Geometry: final body of the model. Coordinates: model frame, mm. A direction names the side the tool comes from. Round coordinates to 2 decimals unless told otherwise and drop trailing zeros. Loops run counter-clockwise (first coordinate to the right, second up) from the corner with the lowest first, then second, coordinate; pieces in that order, holes last. Notation, with made-up numbers: M 76.5,29 L 130.5,29 A15 ccw 130.5,57 Z; hole C 71,58 d4. An arc over 180 degrees is marked long. Answer as a JSON object with one key per item and string values.
Autodesk Fusion 360 part; units mm, degrees
sketch "Sketch1" plane through (0, 0, 0) normal (0, 0, 1) x (1, 0, 0)
  line L0 (7, -22) -> (-7, -22)
  line L1 (-7, -22) -> (-7, 22)
  line L2 (-7, 22) -> (7, 22)
  line L3 (7, 22) -> (7, -22)
  line L4 (7, -22) -> (-7, 22) construction
  line L5 (-7, -22) -> (7, 22) construction
  circle A0 centre (0, 0) radius 3.2483
  circle A1 centre (0, 16) radius 0.75
  circle A2 centre (0, -16) radius 0.75
  dimension "d1" = 1.5
  dimension "d2" = 1.5
extrude "Extrude1" add sketch "Sketch1" along normal blind 13
extrude "Extrude2" add 1 faces at (-2.3333, 22, 4.3333) along direction (0, 1, 0) blind 6
extrude "Extrude3" add 1 faces at (2.3333, -22, 4.3333) along direction (0, -1, 0) blind 6
sketch "Sketch2" plane through (0, 0, 13) normal (0, 0, 1) x (-1, 0, 0)
  circle A0 centre (0, 0) radius 3.2483
  circle A1 centre (0, 16) radius 0.75
  circle A2 centre (0, -16) radius 0.75
  line L0 (7, -28) -> (7, 28)
  line L1 (7, 28) -> (-7, 28)
  line L2 (-7, 28) -> (-7, -28)
  line L3 (-7, -28) -> (7, -28)
sketch "Sketch3" plane through (0, 0, 13) normal (0, 0, 1) x (-1, 0, 0)
  line L0 (7, -28) -> (-7, -28)
  line L1 (-7, -28) -> (-7, -20)
  line L2 (-7, -20) -> (7, -20)
  line L3 (7, -20) -> (7, -28)
  line L4 (7, 20) -> (-7, 20)
  line L5 (-7, 20) -> (-7, 28)
  line L6 (-7, 28) -> (7, 28)
  line L7 (7, 28) -> (7, 20)
extrude "Extrude4" add sketch "Sketch3" along normal blind 11
extrude "Extrude5" add 2 faces at (-2.3333, 25.3333, 24) (-2.3333, -22.6667, 24) along direction (0, 0, 1) blind 9.65
sketch "Sketch4" plane through (7, 0, 0) normal (1, 0, 0) x (0, 1, 0)
  line L0 (-28, 0) -> (28, 0)
  line L1 (28, 0) -> (28, 33.65)
  line L2 (28, 33.65) -> (20, 33.65)
  line L3 (20, 33.65) -> (20, 13)
  line L4 (20, 13) -> (-20, 13)
  line L5 (-20, 13) -> (-20, 33.65)
  line L6 (-20, 33.65) -> (-28, 33.65)
  line L7 (-28, 33.65) -> (-28, 0)
  circle A0 centre (-24.7678, 18.6815) radius 2.0007
  circle A1 centre (24.8, 28.7) radius 2.0005
  dimension "d13" = 4.001
extrude "Extrude6" cut sketch "Sketch4" against normal blind 15 contours A0 | A1
sketch "Sketch5" plane through (-7, 0, 0) normal (-1, 0, 0) x (0, -1, 0)
  circle A0 centre (24.7678, 18.6815) radius 2.0007
  circle A1 centre (-24.8, 28.7) radius 2.0005
  line L0 (-28, 0) -> (28, 0)
  line L1 (28, 0) -> (28, 33.65)
  line L2 (28, 33.65) -> (20, 33.65)
  line L3 (20, 33.65) -> (20, 13)
  line L4 (20, 13) -> (-20, 13)
  line L5 (-20, 13) -> (-20, 33.65)
  line L6 (-20, 33.65) -> (-28, 33.65)
  line L7 (-28, 33.65) -> (-28, 0)
  line L8 (-28, 13) -> (28, 13)
  line L9 (28, 13) -> (28, 35.3728)
  line L10 (28, 35.3728) -> (-28, 35.3728)
  line L11 (-28, 35.3728) -> (-28, 13)
extrude "Extrude7" cut sketch "Sketch5" against normal blind 6 contours L5 L6 L7 L8 L11 | L1 L2 L3 L8 L9
extrude "Extrude8" [suppressed]
extrude "Extrude9" [suppressed]
extrude "Extrude10" [suppressed]
extrude "Extrude11" [suppressed]
1) Reachability of faces 1 (the flat face through (-1, -24, 23)), 2 (the flat face through (3, -20, 23)), 3 (the flat face through (-7, 0, 6)) from +Z, -Z, +X, -X, +Y, -Y: full face, straight path, thin tool, end or side. Return the list, or none.
Results:
{"face 1": "+Z, -X, +Y, -Y", "face 2": "+Z, +X, -X", "face 3": "+Z, -Z, -X, +Y, -Y"}
2) Ray query, line 1 (Y direction, x = 0, z = 3); line 2 (Z direction, x = 4.75, y = 24.8); line 3 (Z direction, x = -3.25, y = 23). Return the intervals inside material, ascending.
Results:
{"line 1": "-28 to -16.75, -15.25 to -3.25, 3.25 to 15.25, 16.75 to 28", "line 2": "0 to 26.7, 30.7 to 33.65", "line 3": "0 to 13"}
3) Section query D-D (z = 5). Return the cut outline in (x, y), and give its area (3 significant figures).
Results:
{"outline": "M -7,-28 L 7,-28 L 7,28 L -7,28 Z; hole C 0,0 d6.5; hole C 0,-16 d1.5; hole C 0,16 d1.5", "area": "747 mm2"}
4) Pull-direction query (X, two-part tool) for faces 4 (the flat face through (-1, 24, 23)), 5 (the cylindrical face through (-0.595, 16.456, 6.409)), 6 (the cylindrical face through (-0.163, -15.268, 6.409)), 7 (the flat face through (1, 28, 13)); classes: +X half, -X half, draft (parallel to the pull), parting line (faces both ways), or undercut.
Results:
{"face 4": "-X half", "face 5": "undercut", "face 6": "undercut", "face 7": "draft"}
5) Section query B-B (y = 24.8). Return the cut outline in (x, z).
Results:
{"outline": "M -7,0 L 7,0 L 7,26.7 L -1,26.7 L -1,13 L -7,13 Z; M -1,30.7 L 7,30.7 L 7,33.65 L -1,33.65 Z"}
6) Section query C-C (x = 1.75). Return the cut outline in (y, z), and give its area (3 significant figures).
Results:
{"outline": "M -28,0 L -2.74,0 L -2.74,13 L -20,13 L -20,33.65 L -28,33.65 Z; M 2.74,0 L 28,0 L 28,33.65 L 20,33.65 L 20,13 L 2.74,13 Z; hole C -24.77,18.68 d4; hole C 24.8,28.7 d4", "area": "962 mm2"}
7) Section query A-A (z = 23.5). Return the cut outline in (x, y), and give its area (3 significant figures).
Results:
{"outline": "M -1,-28 L 7,-28 L 7,-20 L -1,-20 Z; M -1,20 L 7,20 L 7,28 L -1,28 Z", "area": "128 mm2"}
8) Pin query (flat end, axial travel): P1, Ø4.5, axis at y = -24.77, z = 18.68, coming from the -X side; P2, Ø2.5, axis at x = 0, y = 16, coming from the +Z side; P3, Ø7.5, axis at x = 0, y = 0, coming from the -Z side. Return the tip coordinate at first contact, or that it passes through.
Results:
{"P1": "x = -1", "P2": "z = 13", "P3": "z = 0"}
